For this review, use the dimensioned drawing (mm, ordinates from the lowest corner) and the shaded views. Give positions to 0.01 mm unless a question says otherwise; leave off trailing zeros. Order: outer loops, then holes, each group sorted by start corner. A loop starts at its lowest first (then second) coordinate and runs counter-clockwise, first axis right, second up.
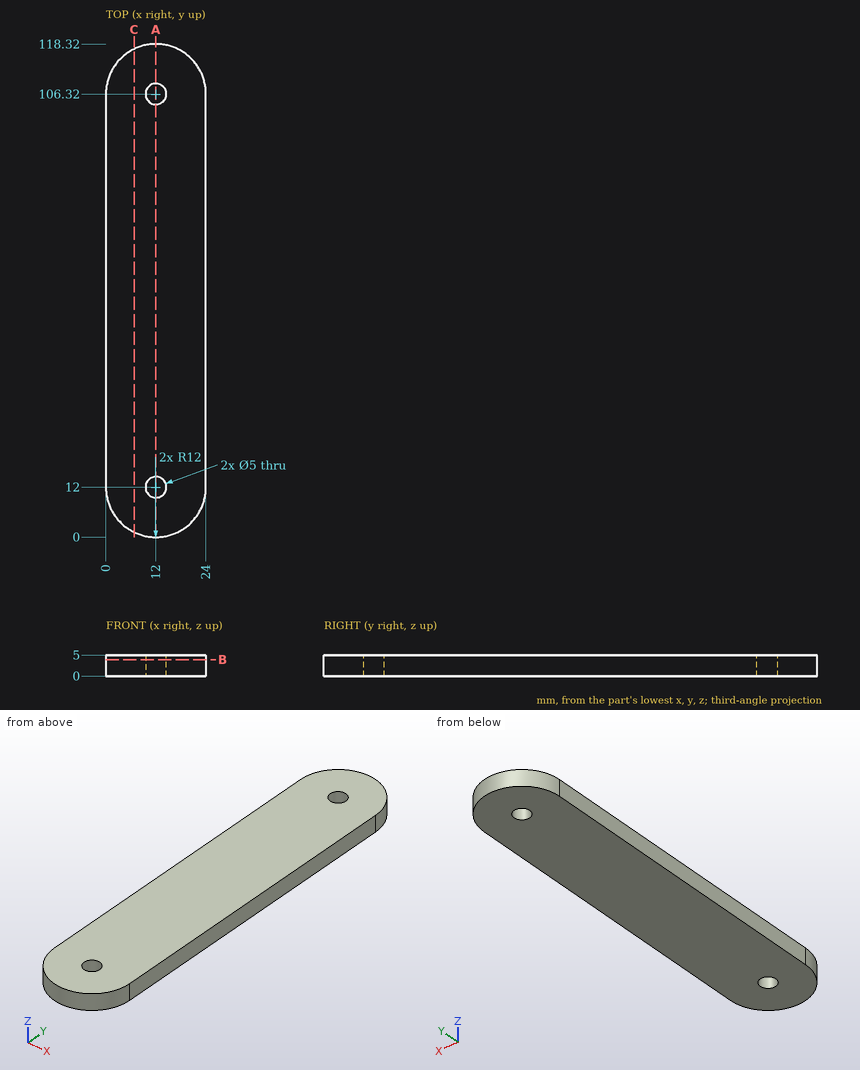
1. To check wall thickness, follow line 1 (Y direction, x = 12, z = 2.15); line 2 (X direction, y = 12, z = 3.6); line 3 (X direction, y = 104.5, z = 3.95). State the ranges of each line that lie inside material, in increasing order.
2. Take a section at B-B (z = 3.9). Write out the cut boundary in (x, y).
3. Insertion check: pin 1 (1.5 mm diameter, centred on x = 4.5, z = 1, fed in from +Y); pin 2 (3 mm diameter, centred on x = 12, y = 106.32, fed in from -Z); pin 3 (3 mm diameter, centred on x = 9, z = 4.5, fed in from -Y). Each pin has a flat end and moves straight along its axis. Give the tip position at first contact, or say it passes through.
4. Take a section at C-C (x = 6.75). Write out the cut boundary in (y, z).
5. Take a section at A-A (x = 12). Write out the cut boundary in (y, z), and give its area (3 significant figures).
Answer:
1. line 1: y = 0 to 9.5, 14.5 to 103.82, 108.82 to 118.32
1. line 2: x = 0 to 9.5, 14.5 to 24
1. line 3: x = 0 to 10.29, 13.71 to 24
2. outline: (0, 12) arc R12 ccw to (24, 12) - (24, 106.32) arc R12 ccw to (0, 106.32) - close; hole circle Ø5 at (12, 12); hole circle Ø5 at (12, 106.32)
3. pin 1: stops at y = 116.24
3. pin 2: passes through
3. pin 3: stops at y = 0.09
4. outline: (1.21, 0) - (117.11, 0) - (117.11, 5) - (1.21, 5) - close
5. outline: (0, 0) - (9.5, 0) - (9.5, 5) - (0, 5) - close; (14.5, 0) - (103.82, 0) - (103.82, 5) - (14.5, 5) - close; (108.82, 0) - (118.32, 0) - (118.32, 5) - (108.82, 5) - close
5. area: 542 mm2
